Part model, mm, in its own coordinate system. A direction names the side the tool comes from. Coordinates: 2 decimals unless noted, no trailing zeros. Loops run counter-clockwise (first coordinate to the right, second up) from the corner with the lowest first, then second, coordinate; pieces in that order, holes last.
Autodesk Inventor part; units mm, degrees
ref_plane "YZ Plane" through (0, 0, 0) normal (1, 0, 0) x (0, 1, 0)
ref_plane "XZ Plane" through (0, 0, 0) normal (0, 1, 0) x (-1, 0, 0)
ref_plane "XY Plane" through (0, 0, 0) normal (0, 0, 1) x (1, 0, 0)
ref_plane "Work Plane1" through (15.4052, 15.0652, 4.9) normal (0, 0, 1) x (0, 1, 0)
sketch "Sketch1" plane through (15.4052, 15.0652, 4.9) normal (0, 0, 1) x (0, 1, 0)
  circle A0 centre (5.7948, 15.4052) radius 2.5
  circle A1 centre (-15.6052, -5.7948) radius 2.5
  line L0 (-20.0856, 39.0762) -> (-20.0856, 40.2052)
  line L1 (-20.0856, 40.2052) -> (-38.2052, 40.2052)
  arc A2 (-38.2052, 40.2052) -> (-40.2052, 38.2052) centre (-38.2052, 38.2052) ccw
  line L2 (-40.2052, 20.2953) -> (-40.2052, 38.2052)
  line L3 (-40.2052, 20.2953) -> (-39.0783, 20.2953)
  arc A3 (-39.0783, 20.2953) -> (-38.6768, 20.6232) centre (-39.0783, 20.7051) ccw
  arc A4 (-34.5391, 20.2052) -> (-38.6768, 20.6232) centre (-36.6291, 20.2052) ccw
  line L4 (-34.5391, 20.2052) -> (-34.5391, 10.4067)
  arc A5 (-38.647, 9.8643) -> (-34.5391, 10.4067) centre (-36.6023, 10.2052) ccw
  line L5 (-38.647, 9.8643) -> (-38.6775, 9.9849)
  arc A6 (-38.6775, 9.9849) -> (-39.0762, 10.3249) centre (-39.083, 9.9131) ccw
  line L6 (-39.0762, 10.3249) -> (-40.2052, 10.3249)
  line L7 (-40.2052, -7.7948) -> (-40.2052, 10.3249)
  arc A7 (-40.2052, -7.7948) -> (-38.2052, -9.7948) centre (-38.2052, -7.7948) ccw
  line L8 (-38.2052, -9.7948) -> (-20.2052, -9.7948)
  line L9 (-20.2052, -9.7948) -> (-20.2052, -10.8453)
  arc A8 (-20.6052, -11.3352) -> (-20.2052, -10.8453) centre (-20.7052, -10.8453) ccw
  arc A9 (-20.6052, -11.3352) -> (-20.2052, -15.2948) centre (-20.2052, -13.2948) ccw
  line L10 (-20.2052, -15.2948) -> (-10.2052, -15.2948)
  arc A10 (-10.2052, -15.2948) -> (-9.8052, -11.3352) centre (-10.2052, -13.2948) ccw
  arc A11 (-10.2052, -10.8453) -> (-9.8052, -11.3352) centre (-9.7052, -10.8453) ccw
  line L11 (-10.2052, -10.8453) -> (-10.2052, -9.7948)
  line L12 (-10.2052, -9.7948) -> (7.7948, -9.7948)
  arc A12 (7.7948, -9.7948) -> (9.7948, -7.7948) centre (7.7948, -7.7948) ccw
  line L13 (9.7948, 10.2052) -> (9.7948, -7.7948)
  line L14 (9.7948, 10.2052) -> (10.8453, 10.2052)
  arc A13 (11.3352, 9.8052) -> (10.8453, 10.2052) centre (10.8453, 9.7052) ccw
  arc A14 (11.3352, 9.8052) -> (15.2948, 10.2052) centre (13.2948, 10.2052) ccw
  line L15 (15.2948, 10.2052) -> (15.2948, 20.2052)
  arc A15 (15.2948, 20.2052) -> (11.3352, 20.6052) centre (13.2948, 20.2052) ccw
  arc A16 (10.8453, 20.2052) -> (11.3352, 20.6052) centre (10.8453, 20.7052) ccw
  line L16 (10.8453, 20.2052) -> (9.7948, 20.2052)
  line L17 (9.7948, 38.2052) -> (9.7948, 20.2052)
  arc A17 (9.7948, 38.2052) -> (7.7948, 40.2052) centre (7.7948, 38.2052) ccw
  line L18 (7.7948, 40.2052) -> (-10.1151, 40.2052)
  line L19 (-10.1151, 40.2052) -> (-10.1151, 39.0783)
  arc A18 (-10.1151, 39.0783) -> (-9.7873, 38.6768) centre (-9.7054, 39.0783) ccw
  arc A19 (-10.2052, 34.5391) -> (-9.7873, 38.6768) centre (-10.2052, 36.6291) ccw
  line L20 (-10.2052, 34.5391) -> (-20.0038, 34.5391)
  arc A20 (-20.5462, 38.647) -> (-20.0038, 34.5391) centre (-20.2052, 36.6023) ccw
  line L21 (-20.5462, 38.647) -> (-20.4256, 38.6775)
  arc A21 (-20.4256, 38.6775) -> (-20.0856, 39.0762) centre (-20.4974, 39.083) ccw
  line L22 (-0.2052, 32.2052) -> (-30.2052, 32.2052)
  arc A22 (1.7948, 30.2052) -> (-0.2052, 32.2052) centre (-0.2052, 30.2052) ccw
  line L23 (1.7948, 30.2052) -> (1.7948, 0.2052)
  arc A23 (-0.2052, -1.7948) -> (1.7948, 0.2052) centre (-0.2052, 0.2052) ccw
  line L24 (-0.2052, -1.7948) -> (-30.2052, -1.7948)
  arc A24 (-32.2052, 0.2052) -> (-30.2052, -1.7948) centre (-30.2052, 0.2052) ccw
  line L25 (-32.2052, 0.2052) -> (-32.2052, 30.2052)
  arc A25 (-30.2052, 32.2052) -> (-32.2052, 30.2052) centre (-30.2052, 30.2052) ccw
  circle A26 centre (-35.2052, 35.2052) radius 2.425
  circle A27 centre (-29.7052, 36.0052) radius 2.65
  circle A28 centre (-36.0052, 29.7052) radius 2.65
  circle A29 centre (-35.2052, -4.7948) radius 2.425
  circle A30 centre (-29.7052, -5.5948) radius 2.65
  circle A31 centre (-36.0052, 0.7052) radius 2.65
  circle A32 centre (4.7948, 35.2052) radius 2.425
  circle A33 centre (-0.7052, 36.0052) radius 2.65
  circle A34 centre (5.5948, 29.7052) radius 2.65
  circle A35 centre (5.5948, 0.7052) radius 2.65
  circle A36 centre (-0.7052, -5.5948) radius 2.65
  circle A37 centre (4.7948, -4.7948) radius 2.425
  point P0 (-15.0652, 15.4052)
extrude "Extrusion1" add sketch "Sketch1" against normal blind 5 draft -1 contours A22 L23 A23 L24 A24 L25 A25 L22
sketch "Sketch2" plane through (15.4052, 15.0652, 4.9) normal (0, 0, 1) x (1, 0, 0)
  circle A0 centre (-26.2552, -7.0652) radius 3
  circle A1 centre (-26.2552, -23.0652) radius 3
  circle A2 centre (-4.2552, -15.0652) radius 1.6
  line L0 (-50.1952, -15.0652) -> (19.3848, -15.0652)
  point P0 (-15.4052, -15.0652)
extrude "Extrusion2" cut sketch "Sketch2" against normal through all
properties part number "30_Cube_Z_Focus_Drylin_NEMA_counterplate"
Q1. Saw through at C-C (x = 11.15). List the corners of the cut face in (y, z).
Q2. Mould opens along Y. For faces 4 (the cylindrical face through (12.676, 0.481, 2.435)), 5 (the flat face through (0, 0, 4.9)), 6 (the cylindrical face through (-7.99, -7.1, 2.44)), 7 (the conical face through (16.57, -16.54, 2.44)) say: released by +Y, released by -Y, zero draft, split by the parting line, or undercut.
Q3. Saw through at B-B (y = 0). List the corners of the cut face in (x, z).
Q4. Probe line 1 (Y direction, x = -12.5, z = 2.9); line 2 (Y direction, x = -10.85, z = 2.8); line 3 (Y direction, x = 11, z = 0.1). List the from-to ranges inside material, lowest first.
Q5. Tool access for faces 1 (the conical face through (16.6, 16.23, 2.44)), 2 (the conical face through (-16.17, 16.26, 2.44)), 3 (the conical face through (-16.2, -16.51, 2.44)): list every direction of +Z, -Z, +X, -X, +Y, -Y with a clear straight run to the whole face (end or side of a thin tool).
Q6. Saw through at A-A (x = -10.85). List the corners of the cut face in (y, z).
Q7. Drop a flat-ended pin along its axis: P1, Ø5, axis at x = -10.85, y = -8, coming from the +Z side. Give the stop position or say it passes through.
Q8. Saw through at D-D (z = 2.65). List the corners of the cut face in (x, y), plus the area to 3 significant figures.
Checked values:
1. outline: (-17.14, 4.9) - (-17.05, -0.1) - (-1.6, -0.1) - (-1.6, 4.9) - close; (1.6, -0.1) - (16.77, -0.1) - (16.86, 4.9) - (1.6, 4.9) - close
2. face 4: undercut
2. face 5: zero draft
2. face 6: undercut
2. face 7: released by -Y
3. outline: (-16.8, 4.9) - (-16.71, -0.1) - (9.55, -0.1) - (9.55, 4.9) - close; (12.75, -0.1) - (17.11, -0.1) - (17.2, 4.9) - (12.75, 4.9) - close
4. line 1: y = -17.11 to -10.51, -5.49 to 5.49, 10.51 to 16.83
4. line 2: y = -17.1 to -11, -5 to 5, 11 to 16.82
4. line 3: y = -17.06 to -1.59, 1.59 to 16.78
5. face 1: -Z, +X, +Y
5. face 2: -Z, -X, +Y
5. face 3: -Z, -X, -Y
6. outline: (-17.14, 4.9) - (-17.05, -0.1) - (-11, -0.1) - (-11, 4.9) - close; (-5, -0.1) - (5, -0.1) - (5, 4.9) - (-5, 4.9) - close; (11, -0.1) - (16.77, -0.1) - (16.86, 4.9) - (11, 4.9) - close
7. P1: passes through
8. outline: (-16.76, -15.14) arc R1.96 ccw to (-14.8, -17.1) - (15.2, -17.1) arc R1.96 ccw to (17.16, -15.14) - (17.16, 14.86) arc R1.96 ccw to (15.2, 16.82) - (-14.8, 16.82) arc R1.96 ccw to (-16.76, 14.86) - close; hole circle Ø6 at (-10.85, -8); hole circle Ø6 at (-10.85, 8); hole circle Ø3.2 at (11.15, 0)
8. area: 1,080 mm2
